Here's how the part is built. I have some questions about the finished solid (model axes, mm). A direction names the side the tool comes from. Coordinates: 2 decimals unless noted, no trailing zeros. Use CSV: the item, a comma, the result in double quotes. Start each with the question number.
Q1. Which directions (+Z, -Z, +X, -X, +Y, -Y) give clear straight access to the entire face, cutting with the end or side of a thin tool? Please do faces 1 (the flat face through (0, -8, 0.5)), 2 (the flat face through (19.883, -24.737, 0.74)), 3 (the flat face through (-15.93, -37.73, 0.74)).
Q2. Please list where these lines run through material, in increasing order: probe 1 along X at (y, z) = (-44.5, 0.75); probe 2 along Y at (x, z) = (-33, 0.5); probe 3 along Y at (x, z) = (-10, 0.55). Write a range as [from, to].
Q3. If we mould it in two halves opening along Y, with no side actions, what happens to faces 4 (the cylindrical face through (9.079, 10.845, 0.74)), 5 (the flat face through (9, -9, 1.5)), 6 (the cylindrical face through (12.07, 12.53, 0.74))? For each: +Y half, -Y half, draft (parallel to the pull), parting line (faces both ways), or undercut.
Q4. If we section it at A-A (z = 1): State how many separate pieces and enclosed holes the cut face has, and give its area (3 significant figures).
Q5. For pin 1 Ø1.3 at (x, y) = (32.67, -35.16) entering from -Z, with a flat end and sliding along its axis, tell me the tip position at first contact or that it passes through.
from build123d import *

# Parameters (mm, degrees)
F0_R     = 0.8
F0_R_2   = 2.5
F0_R_3   = 1.25
F1_DEPTH = 1.5
F3_DEPTH = 1


with BuildPart() as f1:
    # F0 (on Top) → F1 (new body)
    with BuildSketch(Plane.XY):
        with BuildLine():
            Line((-31.716832, 9.520675), (-13.730384, -8.327864))
            ThreePointArc((-13.730384, -8.327864), (-13.294515, -8.974629), (-13.139162, -9.738927))
            ThreePointArc((-13.139162, -9.738927), (-12.767146, -11.505125), (-11.486594, -12.777146))
            ThreePointArc((-11.486594, -12.777146), (-10.714692, -13.512731), (-10.430463, -14.540413))
            Line((-10.430463, -14.540413), (-10.430463, -16.13337))
            ThreePointArc((-10.430463, -16.13337), (-10.746412, -17.473471), (-11.62771, -18.531303))
            Line((-11.62771, -18.531303), (-15.493242, -21.437387))
            Line((-15.493242, -21.437387), (-27.909361, -30.771753))
            ThreePointArc((-27.909361, -30.771753), (-29.655032, -31.614116), (-31.58989, -31.729297))
            ThreePointArc((-31.58989, -31.729297), (-39.836032, -43.215069), (-25.70144, -43.582652))
            ThreePointArc((-25.70144, -43.582652), (-24.79371, -42.416415), (-23.584708, -41.566476))
            Line((-23.584708, -41.566476), (-8.058335, -33.788427))
            ThreePointArc((-8.058335, -33.788427), (-7.655382, -33.419748), (-7.506234, -32.894343))
            Line((-7.506234, -32.894343), (-7.506234, -32.096117))
            Line((-7.506234, -32.096117), (-0.518092, -33.32136))
            ThreePointArc((-0.518092, -33.32136), (0, -33.366435), (0.518092, -33.32136))
            Line((0.518092, -33.32136), (7.506234, -32.096117))
            Line((7.506234, -32.096117), (7.506234, -32.894343))
            ThreePointArc((7.506234, -32.894343), (7.655382, -33.419748), (8.058335, -33.788427))
            Line((8.058335, -33.788427), (23.584708, -41.566476))
            ThreePointArc((23.584708, -41.566476), (24.79371, -42.416415), (25.70144, -43.582652))
            ThreePointArc((25.70144, -43.582652), (39.836032, -43.215069), (31.58989, -31.729297))
            ThreePointArc((31.58989, -31.729297), (29.655032, -31.614116), (27.909361, -30.771753))
            Line((27.909361, -30.771753), (11.62771, -18.531303))
            ThreePointArc((11.62771, -18.531303), (10.746412, -17.473471), (10.430463, -16.13337))
            Line((10.430463, -16.13337), (10.430463, -14.540413))
            ThreePointArc((10.430463, -14.540413), (10.714692, -13.512731), (11.486594, -12.777146))
            ThreePointArc((11.486594, -12.777146), (12.767146, -11.505125), (13.139162, -9.738927))
            ThreePointArc((13.139162, -9.738927), (13.294515, -8.974629), (13.730384, -8.327864))
            Line((13.730384, -8.327864), (31.716832, 9.520675))
            Line((31.716832, 9.520675), (33.960373, 11.747013))
            ThreePointArc((33.960373, 11.747013), (35.545021, 12.807352), (37.411379, 13.197397))
            ThreePointArc((37.411379, 13.197397), (43.844593, 25.794573), (29.811857, 24.017664))
            ThreePointArc((29.811857, 24.017664), (29.04528, 22.667242), (27.901363, 21.617129))
            Line((27.901363, 21.617129), (24.304559, 19.22573))
            Line((24.304559, 19.22573), (14.596146, 12.77092))
            ThreePointArc((14.596146, 12.77092), (12.032551, 12.544056), (10.450405, 14.573909))
            Line((10.450405, 14.573909), (9.220249, 14.583025))
            Line((9.220249, 14.583025), (2.354764, 14.583025))
            ThreePointArc((2.354764, 14.583025), (0, 16.937789), (-2.354764, 14.583025))
            Line((-2.354764, 14.583025), (-9.220249, 14.583025))
            Line((-9.220249, 14.583025), (-10.450405, 14.573909))
            ThreePointArc((-10.450405, 14.573909), (-12.032551, 12.544056), (-14.596146, 12.77092))
            Line((-14.596146, 12.77092), (-24.304559, 19.22573))
            Line((-24.304559, 19.22573), (-27.901363, 21.617129))
            ThreePointArc((-27.901363, 21.617129), (-29.04528, 22.667242), (-29.811857, 24.017664))
            ThreePointArc((-29.811857, 24.017664), (-43.844593, 25.794573), (-37.411379, 13.197397))
            ThreePointArc((-37.411379, 13.197397), (-35.545021, 12.807352), (-33.960373, 11.747013))
            Line((-33.960373, 11.747013), (-31.716832, 9.520675))
        make_face()
        with Locations((-37.171396, -39.655857)):
            Circle(F0_R, mode=Mode.SUBTRACT)
        with Locations((-32.671396, -44.155857)):
            Circle(F0_R, mode=Mode.SUBTRACT)
        with Locations((-32.671396, -39.655857)):
            Circle(F0_R_2, mode=Mode.SUBTRACT)
        with Locations((-28.171396, -39.655857)):
            Circle(F0_R, mode=Mode.SUBTRACT)
        with Locations((-32.671396, -35.155857)):
            Circle(F0_R, mode=Mode.SUBTRACT)
        with Locations((-5.75, -29.833322)):
            Circle(F0_R_3, mode=Mode.SUBTRACT)
        with Locations((-10, -10)):
            Circle(F0_R_3, mode=Mode.SUBTRACT)
        with Locations((5.75, -29.833322)):
            Circle(F0_R_3, mode=Mode.SUBTRACT)
        with Locations((32.671396, -44.155857)):
            Circle(F0_R, mode=Mode.SUBTRACT)
        with Locations((28.171396, -39.655857)):
            Circle(F0_R, mode=Mode.SUBTRACT)
        with Locations((32.671396, -39.655857)):
            Circle(F0_R_2, mode=Mode.SUBTRACT)
        with Locations((37.171396, -39.655857)):
            Circle(F0_R, mode=Mode.SUBTRACT)
        with Locations((32.671396, -35.155857)):
            Circle(F0_R, mode=Mode.SUBTRACT)
        with Locations((10, -10)):
            Circle(F0_R_3, mode=Mode.SUBTRACT)
        with Locations((-36.905747, 16.713716)):
            Circle(F0_R, mode=Mode.SUBTRACT)
        with Locations((-41.780824, 20.804392)):
            Circle(F0_R, mode=Mode.SUBTRACT)
        with Locations((-37.297947, 21.196592)):
            Circle(F0_R_2, mode=Mode.SUBTRACT)
        with Locations((-37.690148, 25.679469)):
            Circle(F0_R, mode=Mode.SUBTRACT)
        with Locations((-32.815071, 21.588793)):
            Circle(F0_R, mode=Mode.SUBTRACT)
        with Locations((-10, 10)):
            Circle(F0_R_3, mode=Mode.SUBTRACT)
        with Locations((0, 14.583025)):
            Circle(F0_R_3, mode=Mode.SUBTRACT)
        with Locations((10, 10)):
            Circle(F0_R_3, mode=Mode.SUBTRACT)
        with Locations((36.905747, 16.713716)):
            Circle(F0_R, mode=Mode.SUBTRACT)
        with Locations((32.815071, 21.588793)):
            Circle(F0_R, mode=Mode.SUBTRACT)
        with Locations((37.297947, 21.196592)):
            Circle(F0_R_2, mode=Mode.SUBTRACT)
        with Locations((41.780824, 20.804392)):
            Circle(F0_R, mode=Mode.SUBTRACT)
        with Locations((37.690148, 25.679469)):
            Circle(F0_R, mode=Mode.SUBTRACT)
        with BuildLine():
            ThreePointArc((-7.506234, -32.894343), (-7.655382, -33.419748), (-8.058335, -33.788427))
            Line((-8.058335, -33.788427), (-0.790004, -35.437413))
            ThreePointArc((-0.790004, -35.437413), (0, -35.525903), (0.790004, -35.437413))
            Line((0.790004, -35.437413), (8.058335, -33.788427))
            ThreePointArc((8.058335, -33.788427), (7.655382, -33.419748), (7.506234, -32.894343))
            Line((7.506234, -32.894343), (7.506234, -32.096117))
            Line((7.506234, -32.096117), (0.518092, -33.32136))
            ThreePointArc((0.518092, -33.32136), (0, -33.366435), (-0.518092, -33.32136))
            Line((-0.518092, -33.32136), (-7.506234, -32.096117))
            Line((-7.506234, -32.096117), (-7.506234, -32.894343))
        make_face()
    extrude(amount=F1_DEPTH)

    # F2 (on face) → F3 (cut)
    with BuildSketch(Plane.XY.offset(1.5)):
        with BuildLine():
            Line((-4.045586, -24.454201), (4.045586, -24.454201))
            ThreePointArc((4.045586, -24.454201), (4.752693, -24.161307), (5.045586, -23.454201))
            Line((5.045586, -23.454201), (5.045586, 7.538364))
            ThreePointArc((5.045586, 7.538364), (4.752693, 8.24547), (4.045586, 8.538364))
            Line((4.045586, 8.538364), (-4.045586, 8.538364))
            ThreePointArc((-4.045586, 8.538364), (-4.752693, 8.24547), (-5.045586, 7.538364))
            Line((-5.045586, 7.538364), (-5.045586, -23.454201))
            ThreePointArc((-5.045586, -23.454201), (-4.752693, -24.161307), (-4.045586, -24.454201))
        make_face()
    extrude(amount=-F3_DEPTH, mode=Mode.SUBTRACT)


solid = f1.part
Results below:
1,face 1,"+Z"
1,face 2,"+Z, -Z, +X"
1,face 3,"+Z, -Z, -Y"
2,probe 1,"[-39.04, -33.39], [-31.95, -26.3], [26.3, 31.95], [33.39, 39.04]"
2,probe 2,"[-47.65, -44.89], [-43.43, -42.13], [-37.18, -35.89], [-34.43, -31.66], [10.79, 20.81], [22.37, 27.94]"
2,probe 3,"[-34.76, -11.25], [-8.75, 8.75], [11.25, 14.58]"
3,face 4,"undercut"
3,face 5,"draft"
3,face 6,"+Y half"
4,separate pieces,"1"
4,enclosed holes,"28"
4,area,"2,640 mm^2"
5,pin 1,"through"
